```python
from build123d import *

# Parameters (mm, degrees)
F1_DEPTH = 7
F2_DEPTH = 7
F3_COUNT = 3


with BuildPart() as f1:
    # F0 (on Top) → F1 (new body)
    with BuildSketch(Plane.XY):
        with BuildLine():
            ThreePointArc((11.9814563539, 19.822065477), (13.3904833189, 23.2093401836), (13.8711614234, 26.8463630714))
            Line((13.8711614234, 26.8463630714), (10.9211614234, 26.8463630714))
            ThreePointArc((10.9211614234, 26.8463630714), (10.6899476462, 24.5977268922), (10.0059822983, 22.4431930958))
            ThreePointArc((10.0059822983, 22.4431930958), (11.0715600581, 21.1912957723), (11.9814563539, 19.822065477))
        make_face()
        with BuildLine():
            Line((10.9211614234, 26.8463630714), (13.8711614234, 26.8463630714))
            ThreePointArc((13.8711614234, 26.8463630714), (-0.1288385766, 40.8463630714), (-14.1288385766, 26.8463630714))
            Line((-14.1288385766, 26.8463630714), (-11.1788385766, 26.8463630714))
            ThreePointArc((-11.1788385766, 26.8463630714), (-0.1288385766, 37.8963630714), (10.9211614234, 26.8463630714))
        make_face()
        with BuildLine():
            Line((-11.1788385766, 26.8463630714), (-14.1288385766, 26.8463630714))
            ThreePointArc((-14.1288385766, 26.8463630714), (-13.6141173472, 23.0850791844), (-12.1078019368, 19.6003685354))
            ThreePointArc((-12.1078019368, 19.6003685354), (-11.2232600764, 20.9861133056), (-10.1809036398, 22.2574102536))
            ThreePointArc((-10.1809036398, 22.2574102536), (-10.9264730154, 24.4982594694), (-11.1788385766, 26.8463630714))
        make_face()
        with BuildLine():
            ThreePointArc((13.8638901362, 12.8469559189), (13.3850110996, 16.4592858558), (11.9814563539, 19.822065477))
            ThreePointArc((11.9814563539, 19.822065477), (11.3223593376, 18.7921674983), (10.5759119571, 17.8237073642))
            ThreePointArc((10.5759119571, 17.8237073642), (11.4068648101, 15.3967409836), (11.6883689483, 12.8469559189))
            ThreePointArc((11.6883689483, 12.8469559189), (11.5000217752, 10.7571071583), (10.9410503341, 8.7346103282))
            ThreePointArc((10.9410503341, 8.7346103282), (11.7016712993, 7.6857588306), (12.3620737952, 6.5710829764))
            ThreePointArc((12.3620737952, 6.5710829764), (13.4832096079, 9.6204239761), (13.8638901362, 12.8469559189))
        make_face()
        with BuildLine():
            ThreePointArc((10.5759119571, 17.8237073642), (11.3223593376, 18.7921674983), (11.9814563539, 19.822065477))
            ThreePointArc((11.9814563539, 19.822065477), (11.0715600581, 21.1912957723), (10.0059822983, 22.4431930958))
            ThreePointArc((10.0059822983, 22.4431930958), (9.4947756455, 21.4160270502), (8.879815604, 20.4474061365))
            ThreePointArc((8.879815604, 20.4474061365), (9.8159198522, 19.1924808087), (10.5759119571, 17.8237073642))
        make_face()
        with BuildLine():
            ThreePointArc((-10.1809036398, 22.2574102536), (-11.2232600764, 20.9861133056), (-12.1078019368, 19.6003685354))
            ThreePointArc((-12.1078019368, 19.6003685354), (-11.4298615634, 18.582775506), (-10.6657163684, 17.6282175746))
            ThreePointArc((-10.6657163684, 17.6282175746), (-9.9310448999, 19.010746625), (-9.0181957741, 20.2826881392))
            ThreePointArc((-9.0181957741, 20.2826881392), (-9.6508788607, 21.239826812), (-10.1809036398, 22.2574102536))
        make_face()
        with BuildLine():
            ThreePointArc((-10.6657163684, 17.6282175746), (-11.4298615634, 18.582775506), (-12.1078019368, 19.6003685354))
            ThreePointArc((-12.1078019368, 19.6003685354), (-13.8612508501, 13.1174639217), (-12.3620737952, 6.5710829764))
            ThreePointArc((-12.3620737952, 6.5710829764), (-11.7016712993, 7.6857588306), (-10.9410503341, 8.7346103282))
            ThreePointArc((-10.9410503341, 8.7346103282), (-11.6827716873, 13.2086386164), (-10.6657163684, 17.6282175746))
        make_face()
        with BuildLine():
            ThreePointArc((-10.4139033154, 3.695012549), (-11.478424483, 5.0717889691), (-12.3620737952, 6.5710829764))
            ThreePointArc((-12.3620737952, 6.5710829764), (-3.3860719771, -13.5843482201), (14, 0))
            ThreePointArc((14, 0), (13.5843482201, 3.3860719771), (12.3620737952, 6.5710829764))
            ThreePointArc((12.3620737952, 6.5710829764), (11.478424483, 5.0717889691), (10.4139033154, 3.695012549))
            ThreePointArc((10.4139033154, 3.695012549), (10.8898147743, 1.8746824217), (11.05, 0))
            ThreePointArc((11.05, 0), (-1.8746824217, -10.8898147743), (-10.4139033154, 3.695012549))
        make_face()
        with BuildLine():
            ThreePointArc((-10.9410503341, 8.7346103282), (-11.7016712993, 7.6857588306), (-12.3620737952, 6.5710829764))
            ThreePointArc((-12.3620737952, 6.5710829764), (-11.478424483, 5.0717889691), (-10.4139033154, 3.695012549))
            ThreePointArc((-10.4139033154, 3.695012549), (-9.9504776126, 4.8052570462), (-9.3690986882, 5.8585399009))
            ThreePointArc((-9.3690986882, 5.8585399009), (-10.2563874539, 7.2412012803), (-10.9410503341, 8.7346103282))
        make_face()
        with BuildLine():
            ThreePointArc((10.4139033154, 3.695012549), (11.478424483, 5.0717889691), (12.3620737952, 6.5710829764))
            ThreePointArc((12.3620737952, 6.5710829764), (11.7016712993, 7.6857588306), (10.9410503341, 8.7346103282))
            ThreePointArc((10.9410503341, 8.7346103282), (10.2563874539, 7.2412012803), (9.3690986882, 5.8585399009))
            ThreePointArc((9.3690986882, 5.8585399009), (9.9504776126, 4.8052570462), (10.4139033154, 3.695012549))
        make_face()
        with BuildLine():
            ThreePointArc((3.9122229389, 13.4422658684), (7.5626502677, 15.1484573034), (10.5759119571, 17.8237073642))
            ThreePointArc((10.5759119571, 17.8237073642), (9.8159198522, 19.1924808087), (8.879815604, 20.4474061365))
            ThreePointArc((8.879815604, 20.4474061365), (-0.0271481286, 15.7968309975), (-9.0181957741, 20.2826881392))
            ThreePointArc((-9.0181957741, 20.2826881392), (-9.9310448999, 19.010746625), (-10.6657163684, 17.6282175746))
            ThreePointArc((-10.6657163684, 17.6282175746), (-7.6557852491, 15.0419116318), (-4.0410615155, 13.404097203))
            ThreePointArc((-4.0410615155, 13.404097203), (-0.0671867283, 13.9998387828), (3.9122229389, 13.4422658684))
        make_face()
        with BuildLine():
            ThreePointArc((10.9410503341, 8.7346103282), (7.7907276234, 11.6320489639), (3.9122229389, 13.4422658684))
            ThreePointArc((3.9122229389, 13.4422658684), (-0.0616518483, 12.8465242886), (-4.0410615155, 13.404097203))
            ThreePointArc((-4.0410615155, 13.404097203), (-7.8464607172, 11.5945269077), (-10.9410503341, 8.7346103282))
            ThreePointArc((-10.9410503341, 8.7346103282), (-10.2563874539, 7.2412012803), (-9.3690986882, 5.8585399009))
            ThreePointArc((-9.3690986882, 5.8585399009), (0, 11.05), (9.3690986882, 5.8585399009))
            ThreePointArc((9.3690986882, 5.8585399009), (10.2563874539, 7.2412012803), (10.9410503341, 8.7346103282))
        make_face()
        with BuildLine():
            ThreePointArc((-4.0410615155, 13.404097203), (-0.0616518483, 12.8465242886), (3.9122229389, 13.4422658684))
            ThreePointArc((3.9122229389, 13.4422658684), (-0.0671867283, 13.9998387828), (-4.0410615155, 13.404097203))
        make_face()
    extrude(amount=F1_DEPTH)

    # F0 (on Top) → F2 (join)
    with BuildSketch(Plane.XY):
        with BuildLine():
            ThreePointArc((11.9814563539, 19.822065477), (13.3904833189, 23.2093401836), (13.8711614234, 26.8463630714))
            Line((13.8711614234, 26.8463630714), (10.9211614234, 26.8463630714))
            ThreePointArc((10.9211614234, 26.8463630714), (10.6899476462, 24.5977268922), (10.0059822983, 22.4431930958))
            ThreePointArc((10.0059822983, 22.4431930958), (11.0715600581, 21.1912957723), (11.9814563539, 19.822065477))
        make_face()
        with BuildLine():
            Line((10.9211614234, 26.8463630714), (13.8711614234, 26.8463630714))
            ThreePointArc((13.8711614234, 26.8463630714), (-0.1288385766, 40.8463630714), (-14.1288385766, 26.8463630714))
            Line((-14.1288385766, 26.8463630714), (-11.1788385766, 26.8463630714))
            ThreePointArc((-11.1788385766, 26.8463630714), (-0.1288385766, 37.8963630714), (10.9211614234, 26.8463630714))
        make_face()
        with BuildLine():
            Line((-11.1788385766, 26.8463630714), (-14.1288385766, 26.8463630714))
            ThreePointArc((-14.1288385766, 26.8463630714), (-13.6141173472, 23.0850791844), (-12.1078019368, 19.6003685354))
            ThreePointArc((-12.1078019368, 19.6003685354), (-11.2232600764, 20.9861133056), (-10.1809036398, 22.2574102536))
            ThreePointArc((-10.1809036398, 22.2574102536), (-10.9264730154, 24.4982594694), (-11.1788385766, 26.8463630714))
        make_face()
        with BuildLine():
            ThreePointArc((13.8638901362, 12.8469559189), (13.3850110996, 16.4592858558), (11.9814563539, 19.822065477))
            ThreePointArc((11.9814563539, 19.822065477), (11.3223593376, 18.7921674983), (10.5759119571, 17.8237073642))
            ThreePointArc((10.5759119571, 17.8237073642), (11.4068648101, 15.3967409836), (11.6883689483, 12.8469559189))
            ThreePointArc((11.6883689483, 12.8469559189), (11.5000217752, 10.7571071583), (10.9410503341, 8.7346103282))
            ThreePointArc((10.9410503341, 8.7346103282), (11.7016712993, 7.6857588306), (12.3620737952, 6.5710829764))
            ThreePointArc((12.3620737952, 6.5710829764), (13.4832096079, 9.6204239761), (13.8638901362, 12.8469559189))
        make_face()
        with BuildLine():
            ThreePointArc((10.5759119571, 17.8237073642), (11.3223593376, 18.7921674983), (11.9814563539, 19.822065477))
            ThreePointArc((11.9814563539, 19.822065477), (11.0715600581, 21.1912957723), (10.0059822983, 22.4431930958))
            ThreePointArc((10.0059822983, 22.4431930958), (9.4947756455, 21.4160270502), (8.879815604, 20.4474061365))
            ThreePointArc((8.879815604, 20.4474061365), (9.8159198522, 19.1924808087), (10.5759119571, 17.8237073642))
        make_face()
        with BuildLine():
            ThreePointArc((-10.1809036398, 22.2574102536), (-11.2232600764, 20.9861133056), (-12.1078019368, 19.6003685354))
            ThreePointArc((-12.1078019368, 19.6003685354), (-11.4298615634, 18.582775506), (-10.6657163684, 17.6282175746))
            ThreePointArc((-10.6657163684, 17.6282175746), (-9.9310448999, 19.010746625), (-9.0181957741, 20.2826881392))
            ThreePointArc((-9.0181957741, 20.2826881392), (-9.6508788607, 21.239826812), (-10.1809036398, 22.2574102536))
        make_face()
        with BuildLine():
            ThreePointArc((-10.6657163684, 17.6282175746), (-11.4298615634, 18.582775506), (-12.1078019368, 19.6003685354))
            ThreePointArc((-12.1078019368, 19.6003685354), (-13.8612508501, 13.1174639217), (-12.3620737952, 6.5710829764))
            ThreePointArc((-12.3620737952, 6.5710829764), (-11.7016712993, 7.6857588306), (-10.9410503341, 8.7346103282))
            ThreePointArc((-10.9410503341, 8.7346103282), (-11.6827716873, 13.2086386164), (-10.6657163684, 17.6282175746))
        make_face()
        with BuildLine():
            ThreePointArc((-10.4139033154, 3.695012549), (-11.478424483, 5.0717889691), (-12.3620737952, 6.5710829764))
            ThreePointArc((-12.3620737952, 6.5710829764), (-3.3860719771, -13.5843482201), (14, 0))
            ThreePointArc((14, 0), (13.5843482201, 3.3860719771), (12.3620737952, 6.5710829764))
            ThreePointArc((12.3620737952, 6.5710829764), (11.478424483, 5.0717889691), (10.4139033154, 3.695012549))
            ThreePointArc((10.4139033154, 3.695012549), (10.8898147743, 1.8746824217), (11.05, 0))
            ThreePointArc((11.05, 0), (-1.8746824217, -10.8898147743), (-10.4139033154, 3.695012549))
        make_face()
        with BuildLine():
            ThreePointArc((-10.9410503341, 8.7346103282), (-11.7016712993, 7.6857588306), (-12.3620737952, 6.5710829764))
            ThreePointArc((-12.3620737952, 6.5710829764), (-11.478424483, 5.0717889691), (-10.4139033154, 3.695012549))
            ThreePointArc((-10.4139033154, 3.695012549), (-9.9504776126, 4.8052570462), (-9.3690986882, 5.8585399009))
            ThreePointArc((-9.3690986882, 5.8585399009), (-10.2563874539, 7.2412012803), (-10.9410503341, 8.7346103282))
        make_face()
        with BuildLine():
            ThreePointArc((10.4139033154, 3.695012549), (11.478424483, 5.0717889691), (12.3620737952, 6.5710829764))
            ThreePointArc((12.3620737952, 6.5710829764), (11.7016712993, 7.6857588306), (10.9410503341, 8.7346103282))
            ThreePointArc((10.9410503341, 8.7346103282), (10.2563874539, 7.2412012803), (9.3690986882, 5.8585399009))
            ThreePointArc((9.3690986882, 5.8585399009), (9.9504776126, 4.8052570462), (10.4139033154, 3.695012549))
        make_face()
    extrude(amount=F2_DEPTH)

    # F3: F1 ×3 about axis
    f3_axis = Axis((0, 0, 0), (0, 0, 1))


with BuildPart() as f1_1:
    add(f1.part)
    for i in range(1, F3_COUNT):
        add(f1.part.rotate(f3_axis, i * 360 / F3_COUNT))


solid = f1_1.part
```
Source: CAD feature listing. Evaluate the final solid. Frame: model axes, mm. Coordinates: 2 decimals unless noted, no trailing zeros. Write each loop counter-clockwise with the first axis right and the second up, starting at its lowest first coordinate (ties: lowest second). Pieces come first, ordered by that corner, then holes. Notation, with made-up numbers: (-27, -31.75) -> (-12, -31.75) arc R34 ccw to (-12, 6.25) -> close; hole circle Ø4 at (64, 45). An arc over 180 degrees is marked (long way). Return JSON: item names as keys, results as strings. Group by question number.
1) Mould query, pull axis X, two halves, no side actions, for faces 1 (the face through (-11, -3, 7)), 2 (the face through (-4.888, -18.805, 3.451)). Classes: +X half, -X half, draft (parallel to the pull), parting line (faces both ways), or undercut.
2) Section query D-D, the plane z = 3. State how many separate pieces and enclosed holes the cut face has, plus the area to 3 significant figures.
3) Section query C-C, the plane x = 33. Return loops of the section in (y, z), plus the area to 3 significant figures.
4) Section query B-B, the plane y = 34.5. Return loops of the section in (x, z).
5) Ray query, line 1 along Y through (x, z) = (2, 2.25); line 2 along X through (y, z) = (4, 3.25); line 3 along X through (y, z) = (-22.5, 4.5). Return the intervals inside material, ascending.
6) Contact query for flat-ended pins moving along their axis: P1, Ø1.5, axis at y = 28.5, z = 1.5, coming from the -X side; P2, Ø2, axis at x = -29, z = 2, coming from the -Y side; P3, Ø4, axis at y = -20, z = 0.5, coming from the +X side. Output: stop coordinate, or through.
7) Section query A-A, the plane x = 1. Return loops of the section in (y, z).
From the geometry:
{
 "1": {"face 1": "draft", "face 2": "undercut"},
 "2": {"separate pieces": "1", "enclosed holes": "10", "area": "1,060 mm²"},
 "3": {"outline": "(-23.42, 0) -> (-18.63, 0) -> (-18.63, 7) -> (-23.42, 7) -> close; (-7.99, 0) -> (-3.2, 0) -> (-3.2, 7) -> (-7.99, 7) -> close", "area": "67.1 mm²"},
 "4": {"outline": "(-11.85, 0) -> (-8.1, 0) -> (-8.1, 7) -> (-11.85, 7) -> close; (7.84, 0) -> (11.59, 0) -> (11.59, 7) -> (7.84, 7) -> close"},
 "5": {"line 1": "-16.86 to -10.87, 10.87 to 16, 37.69 to 40.68", "line 2": "-20.27 to -16.41, -13.42 to -10.3, 10.3 to 13.42, 16.41 to 20.27", "line 3": "-33.94 to -29.64, -16.73 to -12.43, 12.75 to 17.18, 29.45 to 33.88"},
 "6": {"P1": "x = -14.1", "P2": "y = -26.68", "P3": "x = 36.51"},
 "7": {"outline": "(-15.89, 0) -> (-11, 0) -> (-11, 7) -> (-15.89, 7) -> close; (11, 0) -> (15.85, 0) -> (15.85, 7) -> (11, 7) -> close; (37.84, 0) -> (40.8, 0) -> (40.8, 7) -> (37.84, 7) -> close"}
}
